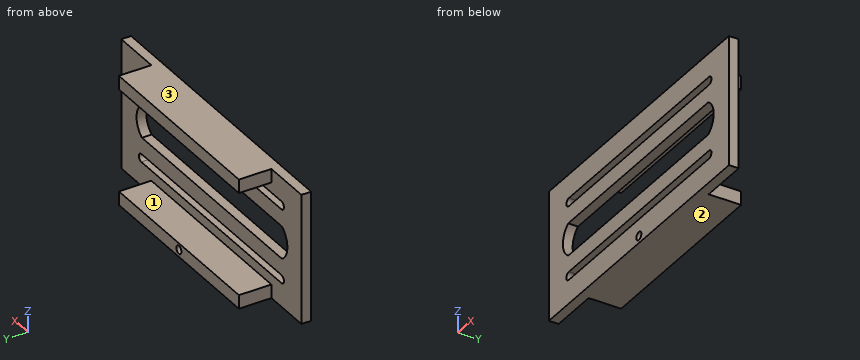
```python
from build123d import *

# Parameters (mm, degrees)
SKETCH2_W           = 228.6
SKETCH2_H           = 101.6
BOSS_EXTRUDE1_DEPTH = 7.62
SKETCH3_W           = 152.4
SKETCH3_H           = 10.668
BOSS_EXTRUDE2_DEPTH = 25.4
CUT_EXTRUDE1_DEPTH  = 8.62
CUT_EXTRUDE2_DEPTH  = 8.62
SKETCH6_R           = 3.175
CUT_EXTRUDE3_DEPTH  = 34.02


with BuildPart() as part:
    # Sketch2 → Boss-Extrude1 (new body)
    with BuildSketch(Plane(origin=(0, 0, 0), x_dir=(1, 0, 0), z_dir=(0, 1, 0))):
        with Locations((114.3, 50.8)):
            Rectangle(SKETCH2_W, SKETCH2_H)
    extrude(amount=BOSS_EXTRUDE1_DEPTH)

    # Sketch3 → Boss-Extrude2 (add)
    with BuildSketch(Plane(origin=(0, 7.62, 0), x_dir=(1, 0, 0), z_dir=(0, 1, 0))):
        with Locations((114.3, 5.334)):
            Rectangle(SKETCH3_W, SKETCH3_H)
        with Locations((114.3, 96.266)):
            Rectangle(SKETCH3_W, SKETCH3_H)
    extrude(amount=BOSS_EXTRUDE2_DEPTH)

    # Sketch4 → Cut-Extrude1 (cut, through all)
    with BuildSketch(Plane(origin=(0, 7.62, 0), x_dir=(1, 0, 0), z_dir=(0, 1, 0))):
        with BuildLine():
            Line((25.4, 24.973599875), (203.2, 24.973599875))
            ThreePointArc((203.2, 24.973599875), (206.375, 21.798599875), (203.2, 18.623599875))
            Line((203.2, 18.623599875), (25.4, 18.623599875))
            ThreePointArc((25.4, 18.623599875), (22.225, 21.798599875), (25.4, 24.973599875))
        make_face()
        with BuildLine():
            Line((25.4, 76.626400125), (203.2, 76.626400125))
            ThreePointArc((203.2, 76.626400125), (206.375, 79.801400125), (203.2, 82.976400125))
            Line((203.2, 82.976400125), (25.4, 82.976400125))
            ThreePointArc((25.4, 82.976400125), (22.225, 79.801400125), (25.4, 76.626400125))
        make_face()
    extrude(amount=-CUT_EXTRUDE1_DEPTH, mode=Mode.SUBTRACT)

    # Sketch5 → Cut-Extrude2 (cut, through all)
    with BuildSketch(Plane(origin=(0, 7.62, 0), x_dir=(1, 0, 0), z_dir=(0, 1, 0))):
        with BuildLine():
            Line((24.632893217, 63.5), (202.432893217, 63.5))
            ThreePointArc((202.432893217, 63.5), (209.248666249, 50.8), (202.432893217, 38.1))
            Line((202.432893217, 38.1), (24.632893217, 38.1))
            ThreePointArc((24.632893217, 38.1), (17.817120184, 50.8), (24.632893217, 63.5))
        make_face()
    extrude(amount=-CUT_EXTRUDE2_DEPTH, mode=Mode.SUBTRACT)

    # Sketch6 → Cut-Extrude3 (cut, through all)
    with BuildSketch(Plane.XZ):
        with Locations((114.3, -96.012)):
            Circle(SKETCH6_R)
    extrude(amount=-CUT_EXTRUDE3_DEPTH, mode=Mode.SUBTRACT)


solid = part.part
```
Part model, mm, in its own coordinate system. Face numbers are marked on the shaded views. Round coordinates to 2 decimals unless told otherwise and drop trailing zeros. Write each loop counter-clockwise with the first axis right and the second up, starting at its lowest first coordinate (ties: lowest second). Pieces come first, ordered by that corner, then holes.
Item 1: Cut at C-C, the plane x = 150.5. Give the cut face in (y, z).
Results:
outline: (0, -101.6) - (33.02, -101.6) - (33.02, -90.93) - (7.62, -90.93) - (7.62, -82.98) - (0, -82.98) - close; (0, -76.63) - (7.62, -76.63) - (7.62, -63.5) - (0, -63.5) - close; (0, -38.1) - (7.62, -38.1) - (7.62, -24.97) - (0, -24.97) - close; (0, -18.62) - (7.62, -18.62) - (7.62, -10.67) - (33.02, -10.67) - (33.02, 0) - (0, 0) - close
Item 2: Cut at A-A, the plane x = 114.3. Give the cut face in (y, z).
Results:
outline: (0, -101.6) - (33.02, -101.6) - (33.02, -99.19) - (0, -99.19) - close; (0, -92.84) - (33.02, -92.84) - (33.02, -90.93) - (7.62, -90.93) - (7.62, -82.98) - (0, -82.98) - close; (0, -76.63) - (7.62, -76.63) - (7.62, -63.5) - (0, -63.5) - close; (0, -38.1) - (7.62, -38.1) - (7.62, -24.97) - (0, -24.97) - close; (0, -18.62) - (7.62, -18.62) - (7.62, -10.67) - (33.02, -10.67) - (33.02, 0) - (0, 0) - close
Item 3: Two-plate mould, pull along Z, no slides. Class the marked faces 1, 2 and 3: +Z half, -Z half, draft (parallel to the pull), parting line (faces both ways), or undercut.
Results:
face 1: undercut
face 2: -Z half
face 3: +Z half
Item 4: Cut at D-D, the plane z = -41.5. Give the cut face in (x, y).
Results:
outline: (0, 0) - (20.98, 0) - (20.98, 7.62) - (0, 7.62) - close; (206.08, 0) - (228.6, 0) - (228.6, 7.62) - (206.08, 7.62) - close
Item 5: Probe L1, parallel to Z at x = 114.3, y = 19; L2, parallel to Z at x = 159.5, y = 6.5; L3, parallel to Z at x = 151, y = 26.5. List the from-to ranges inside material, lowest first.
Results:
L1: z = -101.6 to -99.19, -92.84 to -90.93, -10.67 to 0
L2: z = -101.6 to -82.98, -76.63 to -63.5, -38.1 to -24.97, -18.62 to 0
L3: z = -101.6 to -90.93, -10.67 to 0
Item 6: Drop flat-ended pins along their axis: pin 1 Ø11.5 at (y, z) = (19, -5.5) entering from +X; pin 2 Ø11.5 at (y, z) = (23.5, -6) entering from -X; pin 3 Ø12 at (x, z) = (82.5, -78.5) entering from +Y. Give the stop position or say it passes through.
Results:
pin 1: stops at x = 190.5
pin 2: stops at x = 38.1
pin 3: stops at y = 7.62
Item 7: Cut at B-B, the plane y = 10. Give the cut face in (x, z) (3 decimals).
Results:
outline: (38.1, -101.6) - (190.5, -101.6) - (190.5, -90.932) - (38.1, -90.932) - close; (38.1, -10.668) - (190.5, -10.668) - (190.5, 0) - (38.1, 0) - close; hole circle Ø6.35 at (114.3, -96.012)
